from build123d import *

# Parameters (mm, degrees)
SKETCH1_W                       = 31.15
SKETCH1_H                       = 12.7
SKETCH1_W_2                     = 12.7
SKETCH1_H_2                     = 31.15
BOSS_EXTRUDE1_DEPTH             = 3.175
F_10_32_TAPPED_HOLE1_D          = 4.0386
F_10_32_TAPPED_HOLE1_DEPTH      = 12.7
F_10_32_TAPPED_HOLE1_TIP        = 1.213317848
EDGE_FLANGE1_STRIP_W            = 13.462
EDGE_FLANGE1_STRIP_H            = 3.175
EDGE_FLANGE1_STRIP_CUT_DEPTH    = 27.696197319
EDGE_FLANGE1_RELIEF_W           = 15.0495
EDGE_FLANGE1_RELIEF_H           = 1.5875
EDGE_FLANGE1_RELIEF_CUT_DEPTH   = 3.175
EDGE_FLANGE1_STRIP_2_W          = 13.462
EDGE_FLANGE1_STRIP_2_H          = 3.175
EDGE_FLANGE1_STRIP_CUT_2_DEPTH  = 29.266530926
EDGE_FLANGE1_RELIEF_2_W         = 15.0495
EDGE_FLANGE1_RELIEF_2_H         = 1.5875
EDGE_FLANGE1_RELIEF_CUT_2_DEPTH = 3.175
EDGE_FLANGE1_DEPTH              = 27.696197319
EDGE_FLANGE1_BEND_DEPTH         = 29.266530926


# Sheet-metal steps are written as plain solids
with BuildPart() as part:
    # Sketch1 → Boss-Extrude1 (new body)
    with BuildSketch(Plane.XY):
        with Locations((-21.925, 0)):
            Rectangle(SKETCH1_W, SKETCH1_H)
        Rectangle(SKETCH1_W_2, SKETCH1_H)
        with Locations((0, -21.925)):
            Rectangle(SKETCH1_W_2, SKETCH1_H_2)
        with Locations((21.925, 0)):
            Rectangle(SKETCH1_W, SKETCH1_H)
        with Locations((0, 21.925)):
            Rectangle(SKETCH1_W_2, SKETCH1_H_2)
    extrude(amount=-BOSS_EXTRUDE1_DEPTH)

    # #10-32 Tapped Hole1
    with Locations(Plane.XY):
        with Locations((-17.5, 0), (-32.5, 0), (17.5, 0), (32.5, 0)):
            Hole(F_10_32_TAPPED_HOLE1_D / 2, depth=F_10_32_TAPPED_HOLE1_DEPTH)
            with Locations((0, 0, -(F_10_32_TAPPED_HOLE1_DEPTH + F_10_32_TAPPED_HOLE1_TIP / 2))):  # 118° drill point
                Cone(0, F_10_32_TAPPED_HOLE1_D / 2, F_10_32_TAPPED_HOLE1_TIP, mode=Mode.SUBTRACT)

    # Edge-Flange1 strip (across the edge) → Edge-Flange1 strip cut (cut)
    with BuildSketch(Plane(origin=(6.35, -37.5, 0), x_dir=(-1, 0, 0), z_dir=(0, 1, 0))):
        with Locations((-6.35, -1.5875)):
            Rectangle(EDGE_FLANGE1_STRIP_W, EDGE_FLANGE1_STRIP_H)
    extrude(amount=EDGE_FLANGE1_STRIP_CUT_DEPTH, mode=Mode.SUBTRACT)

    # Edge-Flange1 relief (on the sheet) → Edge-Flange1 relief cut (cut)
    with BuildSketch(Plane(origin=(5.969, -37.5, 0), x_dir=(-1, 0, 0), z_dir=(0, 0, 1))):
        with Locations((-5.93725, -28.489947319)):
            Rectangle(EDGE_FLANGE1_RELIEF_W, EDGE_FLANGE1_RELIEF_H)
    extrude(amount=-EDGE_FLANGE1_RELIEF_CUT_DEPTH, mode=Mode.SUBTRACT)

    # Edge-Flange1 strip 2 (across the edge) → Edge-Flange1 strip cut 2 (cut)
    with BuildSketch(Plane(origin=(-6.35, 37.5, 0), x_dir=(1, 0, 0), z_dir=(0, -1, 0))):
        with Locations((-6.35, -1.5875)):
            Rectangle(EDGE_FLANGE1_STRIP_2_W, EDGE_FLANGE1_STRIP_2_H)
    extrude(amount=EDGE_FLANGE1_STRIP_CUT_2_DEPTH, mode=Mode.SUBTRACT)

    # Edge-Flange1 relief 2 (on the sheet) → Edge-Flange1 relief cut 2 (cut)
    with BuildSketch(Plane(origin=(-5.969, 37.5, 0), x_dir=(1, 0, 0), z_dir=(0, 0, 1))):
        with Locations((-5.93725, -30.060280926)):
            Rectangle(EDGE_FLANGE1_RELIEF_2_W, EDGE_FLANGE1_RELIEF_2_H)
    extrude(amount=-EDGE_FLANGE1_RELIEF_CUT_2_DEPTH, mode=Mode.SUBTRACT)

    # Edge-Flange1 section (across the edge) → Edge-Flange1 (add)
    with BuildSketch(Plane(origin=(6.35, -37.5, 0), x_dir=(-1, 0, 0), z_dir=(0, 1, 0))):
        with BuildLine():
            Line((-3.175, 0.381), (-3.175, 10.756))
            Line((-3.175, 10.756), (0, 10.756))
            Line((0, 10.756), (0, 0.381))
            ThreePointArc((0, 0.381), (0.111592316, 0.111592316), (0.381, 0))
            Line((0.381, 0), (0.381, -3.175))
            ThreePointArc((0.381, -3.175), (-2.133471714, -2.133471714), (-3.175, 0.381))
        make_face()
    extrude(amount=EDGE_FLANGE1_DEPTH)

    # Edge-Flange1 section 2 (across the edge) → Edge-Flange1 bend (add)
    with BuildSketch(Plane(origin=(-6.35, 37.5, 0), x_dir=(1, 0, 0), z_dir=(0, -1, 0))):
        with BuildLine():
            Line((-3.175, 0.381), (-3.175, 10.756))
            Line((-3.175, 10.756), (0, 10.756))
            Line((0, 10.756), (0, 0.381))
            ThreePointArc((0, 0.381), (0.111592316, 0.111592316), (0.381, 0))
            Line((0.381, 0), (0.381, -3.175))
            ThreePointArc((0.381, -3.175), (-2.133471714, -2.133471714), (-3.175, 0.381))
        make_face()
    extrude(amount=EDGE_FLANGE1_BEND_DEPTH)


solid = part.part
Geometry check sheet. Reference: the model listing, model coordinates, mm. A direction names the side the tool comes from. Round coordinates to 2 decimals unless told otherwise and drop trailing zeros. Write each loop counter-clockwise with the first axis right and the second up, starting at its lowest first coordinate (ties: lowest second). Pieces come first, ordered by that corner, then holes.
Item 1: Section check A-A (x = -17.5). Record the boundary of the cut face in (y, z) (3 decimals).
Determined:
outline: (-6.35, -3.175) - (-2.019, -3.175) - (-2.019, 0) - (-6.35, 0) - close; (2.019, -3.175) - (6.35, -3.175) - (6.35, 0) - (2.019, 0) - close
Item 2: Access from +Z, -Z, +X, -X, +Y, -Y to the whole of each face (thin tool, end or side, straight path). Record for faces 5 (the face through (6.35, -7, -2)), 6 (the face through (6.35, -24, 6)), 7 (the face through (6.35, 22, -2)).
Determined:
face 5: +Z, -Z, +X
face 6: +Z, -X, +Y, -Y
face 7: +Z, -Z, +X, +Y
Item 3: Section check B-B (z = 5). Record the boundary of the cut face in (x, y) (3 decimals), plus the area to 3 significant figures.
Determined:
outline: (-9.525, 8.233) - (-6.35, 8.233) - (-6.35, 37.5) - (-9.525, 37.5) - close; (6.35, -37.5) - (9.525, -37.5) - (9.525, -9.804) - (6.35, -9.804) - close
area: 181 mm2
Item 4: Section check C-C (y = 15.5). Record the boundary of the cut face in (x, z) (3 decimals), plus the area to 3 significant figures.
Determined:
outline: (-9.525, 0.381) arc R3.556 ccw to (-5.969, -3.175) - (6.35, -3.175) - (6.35, 0) - (-5.969, 0) arc R0.381 cw to (-6.35, 0.381) - (-6.35, 10.756) - (-9.525, 10.756) - close
area: 81.9 mm2
Item 5: Material ranges on line 1 along Y through (x, z) = (-32.5, -1.9); line 2 along X through (y, z) = (31, 2.5) (3 decimals); line 3 along X through (y, z) = (-9, -1), recorded low to high.
Determined:
line 1: y = -6.35 to -2.02, 2.02 to 6.35
line 2: x = -9.525 to -6.35
line 3: x = -6.35 to 4.38
Item 6: Go/stop test with flat-tipped pins: pin 1 Ø4 at (x, z) = (-6, 5) entering from -Y; pin 2 Ø3 at (y, z) = (-20, 5) entering from +X (3 decimals); pin 3 Ø4.5 at (x, y) = (-32.5, 0) entering from +Z. Record where each tip stops, or that it passes through.
Determined:
pin 1: stops at y = 8.23
pin 2: stops at x = 9.525
pin 3: stops at z = 0
Item 7: Section check D-D (x = 25.5). Record the boundary of the cut face in (y, z) (3 decimals), plus the area to 3 significant figures.
Determined:
outline: (-6.35, -3.175) - (6.35, -3.175) - (6.35, 0) - (-6.35, 0) - close
area: 40.3 mm2
Item 8: Mould release check, pull along Y, two halves, no side actions. Record for faces 1 (the face through (9.525, -24, 5)), 2 (the face through (-5, 6.646, -2)), 3 (the face through (-22, -6.35, -2)), 4 (the face through (22, 6.35, -2)): +Y half, -Y half, draft (parallel to the pull), parting line (faces both ways), or undercut.
Determined:
face 1: draft
face 2: undercut
face 3: -Y half
face 4: +Y half
